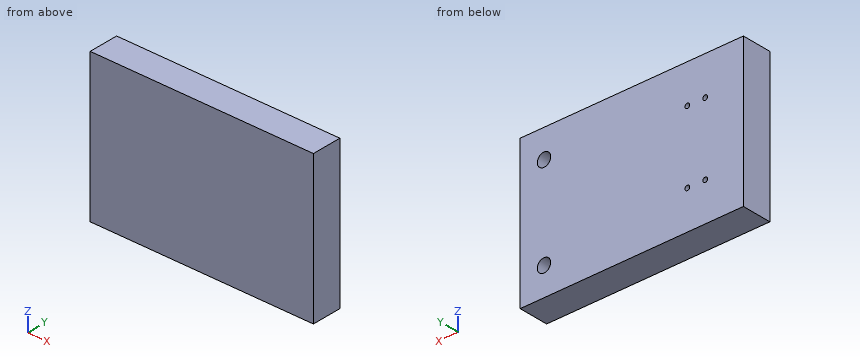
```python
from build123d import *

# Parameters (mm, degrees)
SKETCH2_W             = 75
SKETCH2_H             = 50
PLATE_TOPVIEW_DEPTH   = 10
CHANNEL_DEPTH         = 1
CONNETION_SKETCH_R    = 0.8
CONNETION_SKETCH_R_2  = 2.25
CONNECTING_PORT_DEPTH = 12


with BuildPart() as part:
    # Sketch2 → Plate_topview (new body)
    with BuildSketch(Plane(origin=(0, 0, 0), x_dir=(1, 0, 0), z_dir=(0, 1, 0))):
        Rectangle(SKETCH2_W, SKETCH2_H)
    extrude(amount=PLATE_TOPVIEW_DEPTH)

    # channel_sketch → Channel (cut, symmetric)
    with BuildSketch(Plane(origin=(0, 5, 0), x_dir=(1, 0, 0), z_dir=(0, 1, 0))):
        with BuildLine():
            Line((3.927905037, 0.5), (2.478027018, 2.312347524))
            ThreePointArc((2.478027018, 2.312347524), (2.304186978, 2.450651618), (2.087592613, 2.5))
            Line((2.087592613, 2.5), (-2.43178254, 2.5))
            ThreePointArc((-2.43178254, 2.5), (-2.648376905, 2.450651618), (-2.822216944, 2.312347524))
            Line((-2.822216944, 2.312347524), (-4.272094963, 0.5))
            Line((-4.272094963, 0.5), (-7.964988182, 0.5))
            Line((-7.964988182, 0.5), (-11.943057517, 4.478069335))
            ThreePointArc((-11.943057517, 4.478069335), (-12.024163354, 4.532262522), (-12.119834212, 4.551292639))
            Line((-12.119834212, 4.551292639), (-18.172094963, 4.551292639))
            Line((-18.172094963, 4.551292639), (-18.172094963, 11.492275645))
            ThreePointArc((-18.172094963, 11.492275645), (-18.672094963, 12.801292639), (-19.172094963, 11.492275645))
            Line((-19.172094963, 11.492275645), (-19.172094963, 4.551292639))
            Line((-19.172094963, 4.551292639), (-23.922094963, 4.551292639))
            ThreePointArc((-23.922094963, 4.551292639), (-24.098871659, 4.624515944), (-24.172094963, 4.801292639))
            Line((-24.172094963, 4.801292639), (-24.172094963, 11.492275645))
            ThreePointArc((-24.172094963, 11.492275645), (-24.672094963, 12.801292639), (-25.172094963, 11.492275645))
            Line((-25.172094963, 11.492275645), (-25.172094963, 4.551292639))
            ThreePointArc((-25.172094963, 4.551292639), (-24.879201745, 3.844185858), (-24.172094963, 3.551292639))
            Line((-24.172094963, 3.551292639), (-18.172094963, 3.551292639))
            Line((-18.172094963, 3.551292639), (-12.430494384, 3.551292639))
            Line((-12.430494384, 3.551292639), (-8.879201745, 0))
            Line((-8.879201745, 0), (-12.430494384, -3.551292639))
            Line((-12.430494384, -3.551292639), (-18.172094963, -3.551292639))
            Line((-18.172094963, -3.551292639), (-24.172094963, -3.551292639))
            ThreePointArc((-24.172094963, -3.551292639), (-24.879201745, -3.844185858), (-25.172094963, -4.551292639))
            Line((-25.172094963, -4.551292639), (-25.172094963, -11.492275645))
            ThreePointArc((-25.172094963, -11.492275645), (-24.672094963, -12.801292639), (-24.172094963, -11.492275645))
            Line((-24.172094963, -11.492275645), (-24.172094963, -4.801292639))
            ThreePointArc((-24.172094963, -4.801292639), (-24.098871659, -4.624515944), (-23.922094963, -4.551292639))
            Line((-23.922094963, -4.551292639), (-19.172094963, -4.551292639))
            Line((-19.172094963, -4.551292639), (-19.172094963, -11.492275645))
            ThreePointArc((-19.172094963, -11.492275645), (-18.672094963, -12.801292639), (-18.172094963, -11.492275645))
            Line((-18.172094963, -11.492275645), (-18.172094963, -4.551292639))
            Line((-18.172094963, -4.551292639), (-12.119834212, -4.551292639))
            ThreePointArc((-12.119834212, -4.551292639), (-12.024163354, -4.532262522), (-11.943057517, -4.478069335))
            Line((-11.943057517, -4.478069335), (-7.964988182, -0.5))
            Line((-7.964988182, -0.5), (-4.272094963, -0.5))
            Line((-4.272094963, -0.5), (-2.822216944, -2.312347524))
            ThreePointArc((-2.822216944, -2.312347524), (-2.648376905, -2.450651618), (-2.43178254, -2.5))
            Line((-2.43178254, -2.5), (2.087592613, -2.5))
            ThreePointArc((2.087592613, -2.5), (2.304186978, -2.450651618), (2.478027018, -2.312347524))
            Line((2.478027018, -2.312347524), (3.927905037, -0.5))
            Line((3.927905037, -0.5), (5.077905037, -0.5))
            ThreePointArc((5.077905037, -0.5), (5.254681732, -0.573223305), (5.327905037, -0.75))
            Line((5.327905037, -0.75), (5.327905037, -14.5))
            ThreePointArc((5.327905037, -14.5), (5.620798255, -15.207106781), (6.327905037, -15.5))
            Line((6.327905037, -15.5), (8.327905037, -15.5))
            ThreePointArc((8.327905037, -15.5), (9.035011818, -15.207106781), (9.327905037, -14.5))
            Line((9.327905037, -14.5), (9.327905037, 14.234055176))
            ThreePointArc((9.327905037, 14.234055176), (9.401128341, 14.410831872), (9.577905037, 14.484055176))
            Line((9.577905037, 14.484055176), (11.077905037, 14.484055176))
            ThreePointArc((11.077905037, 14.484055176), (11.254681732, 14.410831872), (11.327905037, 14.234055176))
            Line((11.327905037, 14.234055176), (11.327905037, -14.5))
            ThreePointArc((11.327905037, -14.5), (11.620798255, -15.207106781), (12.327905037, -15.5))
            Line((12.327905037, -15.5), (14.327905037, -15.5))
            ThreePointArc((14.327905037, -15.5), (15.035011818, -15.207106781), (15.327905037, -14.5))
            Line((15.327905037, -14.5), (15.327905037, 14.234055176))
            ThreePointArc((15.327905037, 14.234055176), (15.401128341, 14.410831872), (15.577905037, 14.484055176))
            Line((15.577905037, 14.484055176), (17.077905037, 14.484055176))
            ThreePointArc((17.077905037, 14.484055176), (17.254681732, 14.410831872), (17.327905037, 14.234055176))
            Line((17.327905037, 14.234055176), (17.327905037, -14.5))
            ThreePointArc((17.327905037, -14.5), (17.620798255, -15.207106781), (18.327905037, -15.5))
            Line((18.327905037, -15.5), (20.327905037, -15.5))
            ThreePointArc((20.327905037, -15.5), (21.035011818, -15.207106781), (21.327905037, -14.5))
            Line((21.327905037, -14.5), (21.327905037, -0.75))
            ThreePointArc((21.327905037, -0.75), (21.401128341, -0.573223305), (21.577905037, -0.5))
            Line((21.577905037, -0.5), (24.5, -0.5))
            Line((24.5, -0.5), (24.5, -7))
            ThreePointArc((24.5, -7), (24.646446609, -7.353553391), (25, -7.5))
            Line((25, -7.5), (28.85, -7.5))
            Line((28.85, -7.5), (28.85, -13.55577779))
            ThreePointArc((28.85, -13.55577779), (29.5, -17.55), (30.15, -13.55577779))
            Line((30.15, -13.55577779), (30.15, -7.5))
            Line((30.15, -7.5), (34, -7.5))
            ThreePointArc((34, -7.5), (34.353553391, -7.353553391), (34.5, -7))
            Line((34.5, -7), (34.5, 7))
            ThreePointArc((34.5, 7), (34.353553391, 7.353553391), (34, 7.5))
            Line((34, 7.5), (30.15, 7.5))
            Line((30.15, 7.5), (30.15, 13.55577779))
            ThreePointArc((30.15, 13.55577779), (29.5, 17.55), (28.85, 13.55577779))
            Line((28.85, 13.55577779), (28.85, 7.5))
            Line((28.85, 7.5), (25, 7.5))
            ThreePointArc((25, 7.5), (24.646446609, 7.353553391), (24.5, 7))
            Line((24.5, 7), (24.5, 0.5))
            Line((24.5, 0.5), (21.327905037, 0.5))
            ThreePointArc((21.327905037, 0.5), (20.620798255, 0.207106781), (20.327905037, -0.5))
            Line((20.327905037, -0.5), (20.327905037, -14.25))
            ThreePointArc((20.327905037, -14.25), (20.254681732, -14.426776695), (20.077905037, -14.5))
            Line((20.077905037, -14.5), (18.577905037, -14.5))
            ThreePointArc((18.577905037, -14.5), (18.401128341, -14.426776695), (18.327905037, -14.25))
            Line((18.327905037, -14.25), (18.327905037, 14.484055176))
            ThreePointArc((18.327905037, 14.484055176), (18.035011818, 15.191161957), (17.327905037, 15.484055176))
            Line((17.327905037, 15.484055176), (15.327905037, 15.484055176))
            ThreePointArc((15.327905037, 15.484055176), (14.620798255, 15.191161957), (14.327905037, 14.484055176))
            Line((14.327905037, 14.484055176), (14.327905037, -14.25))
            ThreePointArc((14.327905037, -14.25), (14.254681732, -14.426776695), (14.077905037, -14.5))
            Line((14.077905037, -14.5), (12.577905037, -14.5))
            ThreePointArc((12.577905037, -14.5), (12.401128341, -14.426776695), (12.327905037, -14.25))
            Line((12.327905037, -14.25), (12.327905037, 14.484055176))
            ThreePointArc((12.327905037, 14.484055176), (12.035011818, 15.191161957), (11.327905037, 15.484055176))
            Line((11.327905037, 15.484055176), (9.327905037, 15.484055176))
            ThreePointArc((9.327905037, 15.484055176), (8.620798255, 15.191161957), (8.327905037, 14.484055176))
            Line((8.327905037, 14.484055176), (8.327905037, -14.25))
            ThreePointArc((8.327905037, -14.25), (8.254681732, -14.426776695), (8.077905037, -14.5))
            Line((8.077905037, -14.5), (6.577905037, -14.5))
            ThreePointArc((6.577905037, -14.5), (6.401128341, -14.426776695), (6.327905037, -14.25))
            Line((6.327905037, -14.25), (6.327905037, -0.5))
            ThreePointArc((6.327905037, -0.5), (6.035011818, 0.207106781), (5.327905037, 0.5))
            Line((5.327905037, 0.5), (3.927905037, 0.5))
        make_face()
    extrude(amount=CHANNEL_DEPTH, both=True, mode=Mode.SUBTRACT)

    # connetion_sketch → Connecting_port (cut)
    with BuildSketch(Plane(origin=(0, 5, 0), x_dir=(1, 0, 0), z_dir=(0, 1, 0))):
        with Locations(Location((-24.672094963, 12.051292639, 0), (0, 0, 231.317812547))):
            Circle(CONNETION_SKETCH_R)
        with Locations(Location((-18.672094963, 12.051292639, 0), (0, 0, 231.317812547))):
            Circle(CONNETION_SKETCH_R)
        with Locations(Location((-18.672094963, -12.051292639, 0), (0, 0, 51.317812547))):
            Circle(CONNETION_SKETCH_R)
        with Locations(Location((-24.672094963, -12.051292639, 0), (0, 0, 51.317812547))):
            Circle(CONNETION_SKETCH_R)
        with Locations(Location((29.5, 15.5, 0), (0, 0, 286.791447115))):
            Circle(CONNETION_SKETCH_R_2)
        with Locations(Location((29.5, -15.5, 0), (0, 0, 106.791447115))):
            Circle(CONNETION_SKETCH_R_2)
    extrude(amount=CONNECTING_PORT_DEPTH, mode=Mode.SUBTRACT)


solid = part.part
```
Check sheet for the modelled part. Datum: model origin and axes. Units: mm. Give positions to 0.01 mm unless a question says otherwise; leave off trailing zeros. Write each loop counter-clockwise with the first axis right and the second up, starting at its lowest first coordinate (ties: lowest second). Pieces come first, ordered by that corner, then holes.
Item 1: Gauge pin test, flat ends, axial feed: pin 1 (1.5 mm diameter, centred on x = 19, z = 13, fed in from -Y); pin 2 (3.5 mm diameter, centred on x = 29.5, z = 15.5, fed in from +Y). Record the tip position at first contact, or that the pin passes through.
Item 2: Scan lines: L1, parallel to X at y = 9.75, z = -15.5; L2, parallel to Y at x = -25, z = 11.5; L3, parallel to X at y = 7.25, z = 13.5. Record each from-to range of solid material in increasing order.
Item 3: Cross-section at A-A (x = 26). Enter the section's corners in (y, z).
Item 4: Cross-section at B-B (z = -9). Count the separate pieces of the cut face and the enclosed holes in it, and give its area (3 significant figures).
Report:
1. pin 1: stops at y = 0
1. pin 2: stops at y = 4
2. L1: x = -37.5 to 27.25, 31.75 to 37.5
2. L2: y = 0 to 4
2. L3: x = -37.5 to 28.47, 30.53 to 37.5
3. outline: (0, -25) - (10, -25) - (10, 25) - (0, 25) - close; hole (4, -7.5) - (6, -7.5) - (6, 7.5) - (4, 7.5) - close
4. separate pieces: 1
4. enclosed holes: 7
4. area: 735 mm2
